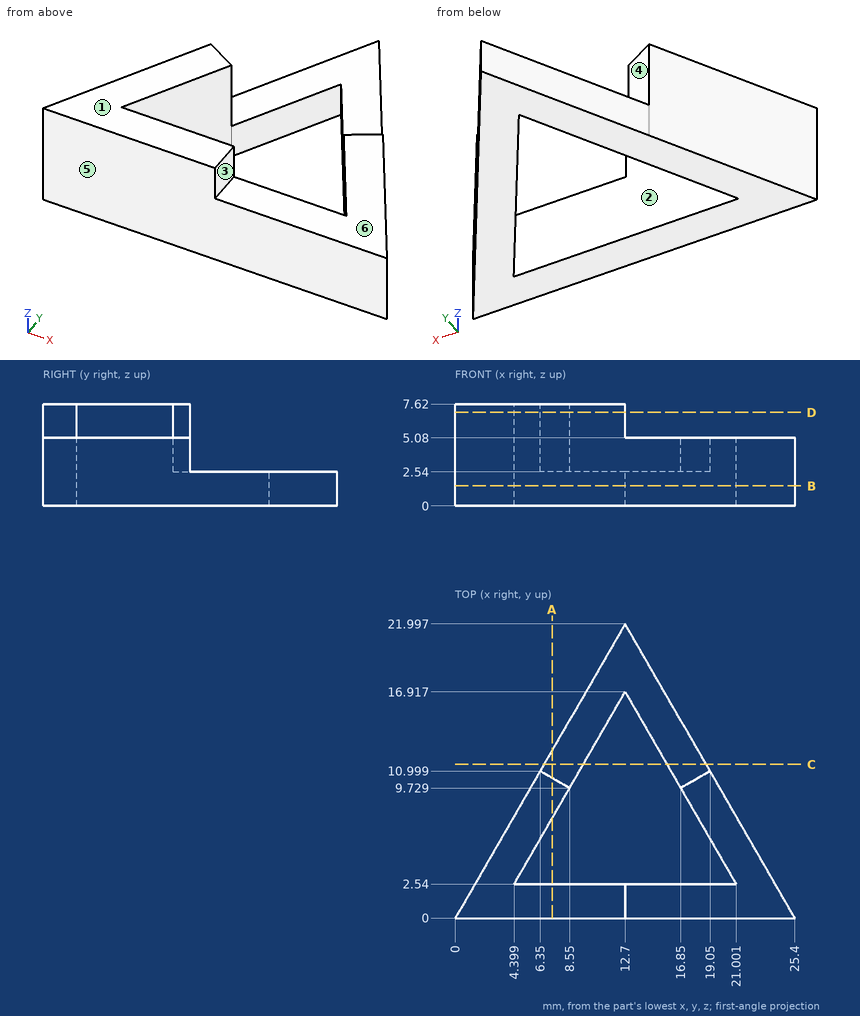
Input: dimensioned drawing with shaded views. Units: mm. Origin: part minimum x, y, z. A direction names the side the tool comes from. Give positions to 0.01 mm unless a question says otherwise; leave off trailing zeros. Write each loop counter-clockwise with the first axis right and the second up, starting at its lowest first coordinate (ties: lowest second). Pieces come first, ordered by that corner, then holes.
Q1. Section C-C, the plane y = 11.5. Output: boundary loops of the cut face in (x, z).
Q2. Set-up query: the marked faces 5 and 6. Return all of +Z, -Z, +X, -X, +Y, -Y with unobstructed straight access to the full face (end or side cutting, diameter ignored); none if empty.
Q3. Section A-A, the plane x = 7.25. Output: boundary loops of the cut face in (y, z).
Q4. Pull-direction query (X, two-part tool) for the marked faces 1, 2, 3 and 4; classes: pulls with the +X half, pulls with the -X half, needs draft (parallel to the pull), parting line crosses it, or undercut.
Q5. Material intervals for probe 1 along Z at (x, y) = (12, 19.25); probe 2 along Z at (x, y) = (14.75, 2.5); probe 3 along Y at (x, z) = (19, 3) (1 decimal), sorted ascending.
Q6. Section B-B, the plane z = 1.5. Output: boundary loops of the cut face in (x, y).
Q7. Section D-D, the plane z = 7. Output: boundary loops of the cut face in (x, y).
Q8. First-contact query: P1, Ø2, axis at y = 1, z = 6.5, coming from the +X side; P2, Ø4, axis at x = 17, z = 5.5, coming from the +Y side (1 decimal); P3, Ø6, axis at x = 14.5, y = 15, coming from the +Z side; P4, Ø2, axis at y = 13, z = 5.5, coming from the -X side. Flat tips, straight axial feed; report the tip coordinate or a pass-through.
Filled in:
1. outline: (6.64, 0) - (9.57, 0) - (9.57, 2.54) - (6.64, 2.54) - close; (15.83, 0) - (18.76, 0) - (18.76, 2.54) - (15.83, 2.54) - close
2. face 5: +Z, -Z, +X, -X, -Y
2. face 6: +Z, +X, +Y, -Y
3. outline: (0, 0) - (2.54, 0) - (2.54, 7.62) - (0, 7.62) - close; (7.48, 0) - (12.56, 0) - (12.56, 2.54) - (10.48, 2.54) - (10.48, 7.62) - (7.48, 7.62) - close
4. face 1: needs draft
4. face 2: undercut
4. face 3: pulls with the +X half
4. face 4: undercut
5. probe 1: z = 0 to 2.54
5. probe 2: z = 0 to 5.08
5. probe 3: y = 0 to 2.5, 6 to 11
6. outline: (0, 0) - (25.4, 0) - (12.7, 22) - close; hole (4.4, 2.54) - (21, 2.54) - (16.85, 9.73) - (12.7, 16.92) - close
7. outline: (0, 0) - (12.7, 0) - (12.7, 2.54) - (4.4, 2.54) - (8.55, 9.73) - (6.35, 11) - close
8. P1: stops at x = 12.7
8. P2: stops at y = 10.9
8. P3: stops at z = 2.54
8. P4: passes through
